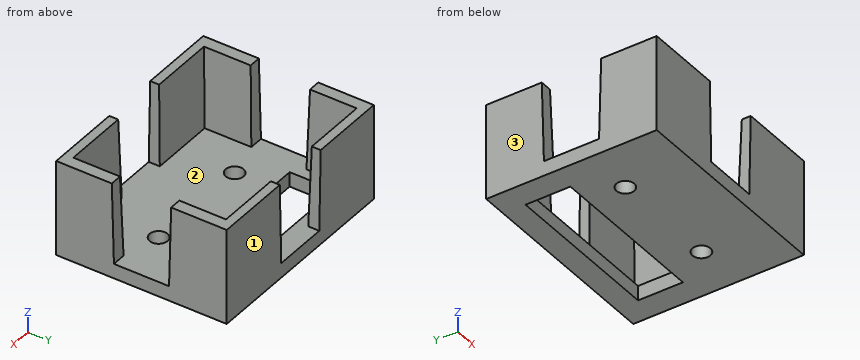
from build123d import *

# Parameters (mm, degrees)
SKETCH2_W           = 36.83
SKETCH2_H           = 29.464
SKETCH2_R           = 1.55
SKETCH2_W_2         = 28.194
SKETCH2_H_2         = 7.747
BOSS_EXTRUDE1_DEPTH = 16.51
CUT_EXTRUDE1_START  = 2.54
SKETCH2_5_W         = 32.004
SKETCH2_5_H         = 25.654
SKETCH2_5_R         = 1.55
SKETCH2_5_W_2       = 28.194
SKETCH2_5_H_2       = 7.747
SKETCH2_5_W_3       = 2.413
SKETCH2_5_H_3       = 9.525
SKETCH2_5_W_4       = 9.525
SKETCH2_5_H_4       = 1.905
CUT_EXTRUDE1_DEPTH  = 14.97
CUT_EXTRUDE1_TAPER  = -1.5


with BuildPart() as part:
    # Sketch2 → Boss-Extrude1 (new body)
    with BuildSketch(Plane.XY):
        Rectangle(SKETCH2_W, SKETCH2_H)
        with Locations((-9.525, -3.175)):
            Circle(SKETCH2_R, mode=Mode.SUBTRACT)
        with Locations((9.525, -3.175)):
            Circle(SKETCH2_R, mode=Mode.SUBTRACT)
        with Locations((0, 7.0485)):
            Rectangle(SKETCH2_W_2, SKETCH2_H_2, mode=Mode.SUBTRACT)
    extrude(amount=BOSS_EXTRUDE1_DEPTH)

    # Sketch2<5> → Cut-Extrude1 (cut, through all)
    with BuildSketch(Plane.XY.offset(CUT_EXTRUDE1_START)):
        Rectangle(SKETCH2_5_W, SKETCH2_5_H)
        with Locations((9.525, -3.175)):
            Circle(SKETCH2_5_R, mode=Mode.SUBTRACT)
        with Locations((-9.525, -3.175)):
            Circle(SKETCH2_5_R, mode=Mode.SUBTRACT)
        with Locations((0, 7.0485)):
            Rectangle(SKETCH2_5_W_2, SKETCH2_5_H_2, mode=Mode.SUBTRACT)
        with Locations((17.2085, 0)):
            Rectangle(SKETCH2_5_W_3, SKETCH2_5_H_3)
        with Locations((0, -13.7795)):
            Rectangle(SKETCH2_5_W_4, SKETCH2_5_H_4)
        with Locations((-17.2085, 0)):
            Rectangle(SKETCH2_5_W_3, SKETCH2_5_H_3)
        with Locations((0, 13.7795)):
            Rectangle(SKETCH2_5_W_4, SKETCH2_5_H_4)
    extrude(amount=CUT_EXTRUDE1_DEPTH, taper=CUT_EXTRUDE1_TAPER, mode=Mode.SUBTRACT)


solid = part.part
The listing builds one solid part. Answer for the finished solid, in the listing's coordinates (mm). Face numbers are marked on the shaded views. Give positions to 0.01 mm unless a question says otherwise; leave off trailing zeros. Order: outer loops, then holes, each group sorted by start corner. A loop starts at its lowest first (then second) coordinate and runs counter-clockwise, first axis right, second up. Notation, with made-up numbers: (13.5, 55.5) - (30.5, 55.5) arc R27 ccw to (30.5, 87.5) - close; hole circle Ø9 at (-8, 6.25). An arc over 180 degrees is marked (long way). Use one line per item in the form item = value.
1) Consider probe 1 along Y at (x, z) = (-1, 2.5) (3 decimals); probe 2 along Y at (x, z) = (9, 2.75); probe 3 along X at (y, z) = (5.75, 1.75) (3 decimals). Determine where each line is inside the solid, lowest interval first. Write a range as [from, to].
Verdict:
probe_1 = [-14.732, 3.175], [10.922, 14.732]
probe_2 = [-14.73, -12.83], [12.83, 14.73]
probe_3 = [-18.415, -14.097], [14.097, 18.415]
2) Find section A-A on x = -3. Determine the outline of the cut face in (y, z) (3 decimals).
Verdict:
outline = (-14.732, 0) - (3.175, 0) - (3.175, 2.54) - (-14.732, 2.54) - close; (10.922, 0) - (14.732, 0) - (14.732, 2.54) - (10.922, 2.54) - close
3) Find section B-B on y = -4.25. Determine the outline of the cut face in (x, z) (3 decimals).
Verdict:
outline = (-18.415, 0) - (-10.642, 0) - (-10.642, 2.54) - (-18.415, 2.54) - close; (-8.408, 0) - (8.408, 0) - (8.408, 2.54) - (-8.408, 2.54) - close; (10.642, 0) - (18.415, 0) - (18.415, 2.54) - (10.642, 2.54) - close
4) Find section C-C on z = 6.75. Give the number of separate pieces and of enclosed holes in the cut face, and give its area (3 significant figures).
Verdict:
separate_pieces = 4
enclosed_holes = 0
area = 172 mm^2
5) The mould has two halves that part along X. Classify the marked faces 1, 2 and 3: released by +X, released by -X, zero draft, split by the parting line, or undercut.
Verdict:
face_1 = zero draft
face_2 = undercut
face_3 = released by -X
